```python
from build123d import *

# Parameters (mm, degrees)
F2_R     = 37.5
F2_R_2   = 33.25
F2_R_3   = 27.25
F3_DEPTH = 22
F4_DEPTH = 11
F5_R     = 1


# Not quite as in the source:
# - a feature of the source that left no trace in its solid (it failed there, or was rolled back) is left out


with BuildPart() as f3:
    # F2 (on Top) → F3 (new body)
    with BuildSketch(Plane.XY):
        Circle(F2_R)
        Circle(F2_R_2, mode=Mode.SUBTRACT)
        Circle(F2_R_2)
        Circle(F2_R_3, mode=Mode.SUBTRACT)
    extrude(amount=F3_DEPTH)

    # F2 (on Top) → F4 (cut)
    with BuildSketch(Plane.XY):
        Circle(F2_R_2)
        Circle(F2_R_3, mode=Mode.SUBTRACT)
    extrude(amount=F4_DEPTH, mode=Mode.SUBTRACT)

    # F5
    f5_edges = [f3.edges().sort_by_distance(p)[0] for p in [
        (-37.5, 0, 22),
        (-27.25, 0, 22),
        (-37.5, 0, 0),
    ]]
    fillet(f5_edges, radius=F5_R)


solid = f3.part
```
For this review, take the finished solid that the model builds, in its own axes (mm). A direction names the side the tool comes from. Round coordinates to 2 decimals unless told otherwise and drop trailing zeros. Write each loop counter-clockwise with the first axis right and the second up, starting at its lowest first coordinate (ties: lowest second). Pieces come first, ordered by that corner, then holes. Notation, with made-up numbers: (1.25, -18) -> (60.25, -18) arc R13 ccw to (60.25, -4) -> close; hole circle Ø3 at (-24.75, -13). An arc over 180 degrees is marked (long way). One line per question, with ' | ' between items. Start each with the question number.
1) Add section A-A (x = 0). Write out the cut boundary in (y, z).
2) Mouldability with a two-part tool opening along Y and no side actions: class faces 1 (the cylindrical face through (-21.625, -16.581, 15.93)), 2 (the cylindrical face through (-4.88, 37.18, 10.86)), 3 (the flat face through (30, -16, 0)), 4 (the flat face through (-5, 27, 11)) as +Y half, -Y half, draft (parallel to the pull), parting line (faces both ways), or undercut.
3) Wall thickness on line 1 along Y through (x, z) = (0, 16.75); line 2 along Y through (x, z) = (0, 4); line 3 along X through (y, z) = (18, 20): over which ranges is each line inside the solid? List them lowest first.
4) For pin 1 Ø3 at (x, z) = (5, 3) entering from -Y; pin 2 Ø1 at (x, z) = (18.5, 11.5) entering from +Y; pin 3 Ø8 at (x, z) = (-2.5, 3.5) entering from -Y, all flat-tipped, find the tip position at first contact; note any pin that passes through.
5) Machinability: for faces 5 (the flat face through (18.8, -21.5, 22)), 6 (the cylindrical face through (17.87, 28.04, 5.42)), which of the approach directions +Z, -Z, +X, -X, +Y, -Y give a long, thin tool a straight path to every point of the face, cutting with its end or side? Answer none if there is none.
6) Add section C-C (z = 15.75). Write out the cut boundary in (x, y), and give its area (3 significant figures).
Reported:
1) outline: (-37.5, 1) arc R1 ccw to (-36.5, 0) -> (-33.25, 0) -> (-33.25, 11) -> (-27.25, 11) -> (-27.25, 21) arc R1 ccw to (-28.25, 22) -> (-36.5, 22) arc R1 ccw to (-37.5, 21) -> close; (27.25, 11) -> (33.25, 11) -> (33.25, 0) -> (36.5, 0) arc R1 ccw to (37.5, 1) -> (37.5, 21) arc R1 ccw to (36.5, 22) -> (28.25, 22) arc R1 ccw to (27.25, 21) -> close
2) face 1: undercut | face 2: parting line | face 3: draft | face 4: undercut
3) line 1: y = -37.5 to -27.25, 27.25 to 37.5 | line 2: y = -37.5 to -33.25, 33.25 to 37.5 | line 3: x = -32.9 to -20.46, 20.46 to 32.9
4) pin 1: stops at y = -37.34 | pin 2: stops at y = 32.9 | pin 3: stops at y = -37.5
5) face 5: +Z, +X, -X, +Y, -Y | face 6: -Z
6) outline: circle Ø75 at (0, 0); hole circle Ø54.5 at (0, 0) | area: 2,090 mm²
